```python
from build123d import *

# Parameters (mm, degrees)
F1_R     = 6
F1_R_2   = 3
F2_DEPTH = 1
F3_R     = 0.2


with BuildPart() as f2:
    # F1 (on offset) → F2 (new body)
    with BuildSketch(Plane.XY):
        Circle(F1_R)
        Circle(F1_R_2, mode=Mode.SUBTRACT)
    extrude(amount=F2_DEPTH)

    # F3
    f3_edges = [f2.edges().sort_by_distance(p)[0] for p in [
        (6, 0, 0.5),
        (-6, 0, 0),
        (-6, 0, 1),
        (-3, 0, 0),
        (-3, 0, 1),
    ]]
    fillet(f3_edges, radius=F3_R)


solid = f2.part
```
CAD build for the part. Positions are in the model's coordinates, mm. Round coordinates to 2 decimals unless told otherwise and drop trailing zeros. Loops run counter-clockwise (first coordinate to the right, second up) from the corner with the lowest first, then second, coordinate; pieces in that order, holes last. Notation, with made-up numbers: (49, 0.5) - (59, 0.5) arc R15 cw to (59, 21.5) - close; hole circle Ø2 at (53.25, -35). An arc over 180 degrees is marked (long way). Return JSON: item names as keys, results as strings. Group by question number.
Q1. Drill centre lines: line 1 along Y through (x, z) = (0, 0.8); line 2 along Y through (x, z) = (-1, 0.55); line 3 along X through (y, z) = (0.75, 0.4). Where is each one in solid material? Low to high. Write a range as [from, to].
Q2. Band-saw the part on B-B on z = 0.65. Give the cut face in (x, y), plus the area to 3 significant figures.
Q3. Two-plate mould, pull along Y, no slides. Class faces 1 (the face through (-3, 0.1, 0.5)), 2 (the face through (2.5, -2.5, 0)), 3 (the face through (-5.994, 0.264, 0.496)): +Y half, -Y half, draft (parallel to the pull), parting line (faces both ways), or undercut.
Q4. Band-saw the part on A-A on x = 0. Give the cut face in (y, z), plus the area to 3 significant figures.
Solutions:
{
 "1": {"line 1": "y = [-6, -3], [3, 6]", "line 2": "y = [-5.92, -2.83], [2.83, 5.92]", "line 3": "x = [-5.95, -2.9], [2.9, 5.95]"},
 "2": {"outline": "circle Ø12 at (0, 0); hole circle Ø6 at (0, 0)", "area": "84.8 mm^2"},
 "3": {"face 1": "undercut", "face 2": "draft", "face 3": "parting line"},
 "4": {"outline": "(-6, 0.2) arc R0.2 ccw to (-5.8, 0) - (-3.2, 0) arc R0.2 ccw to (-3, 0.2) - (-3, 0.8) arc R0.2 ccw to (-3.2, 1) - (-5.8, 1) arc R0.2 ccw to (-6, 0.8) - close; (3, 0.2) arc R0.2 ccw to (3.2, 0) - (5.8, 0) arc R0.2 ccw to (6, 0.2) - (6, 0.8) arc R0.2 ccw to (5.8, 1) - (3.2, 1) arc R0.2 ccw to (3, 0.8) - close", "area": "5.93 mm^2"}
}
